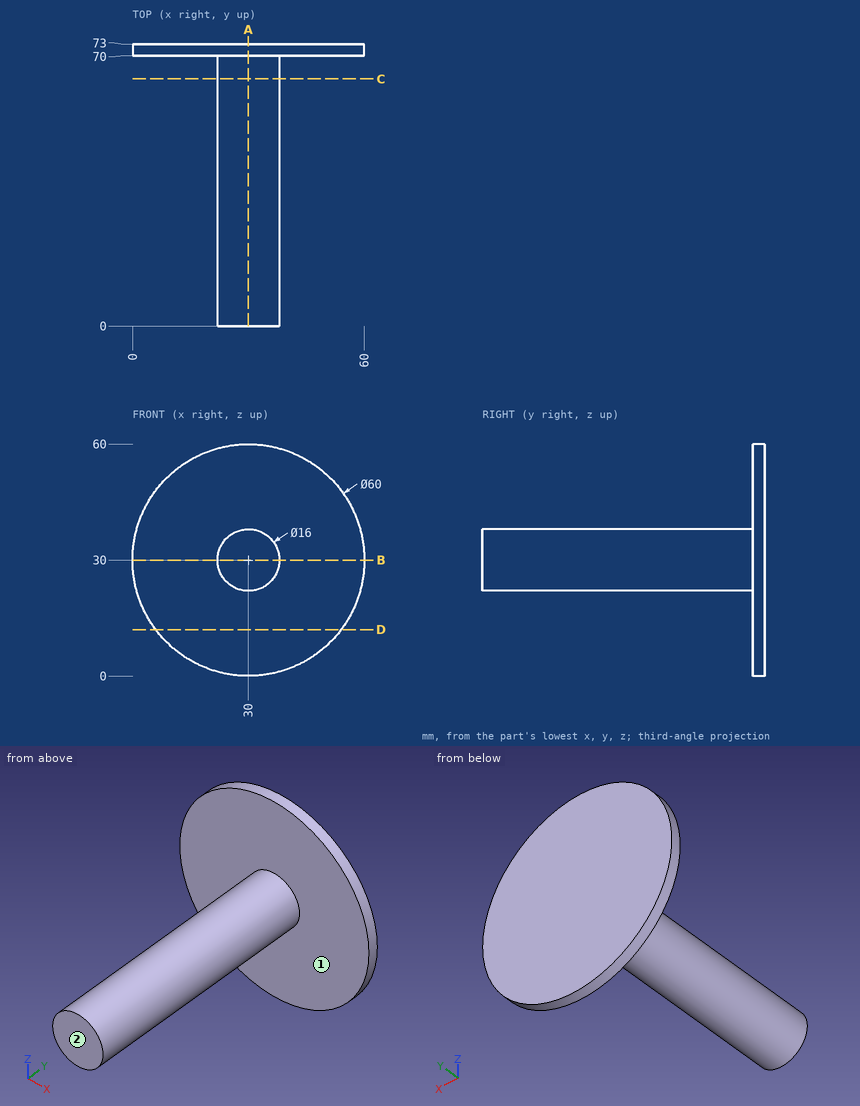
Geometry: see drawing. Coordinates: mm, zero at the bounding-box minimum. A direction names the side the tool comes from. Give positions to 0.01 mm unless a question says otherwise; leave off trailing zeros. Order: outer loops, then holes, each group sorted by start corner. A loop starts at its lowest first (then second) coordinate and runs counter-clockwise, first axis right, second up. Notation, with made-up numbers: (-29.5, 79.5) - (-15.5, 79.5) arc R9 ccw to (-15.5, 94.5) - close; hole circle Ø4 at (-35.75, 70.25). An arc over 180 degrees is marked (long way). Use a Markdown table: item, result.
(1) Section query B-B (z = 30). Output: boundary loops of the cut face in (x, y), then the cut area to 3 significant figures.
Computed values:
| item | result |
|---|---|
| outline | (0, 70) - (22, 70) - (22, 0) - (38, 0) - (38, 70) - (60, 70) - (60, 73) - (0, 73) - close |
| area | 1,300 mm2 |
(2) Pin query (flat end, axial travel): pin 1 (6 mm diameter, centred on x = 37.5, y = 50.5, fed in from +Z); pin 2 (3 mm diameter, centred on y = 38.5, z = 26.5, fed in from +X); pin 3 (10 mm diameter, centred on x = 39.5, y = 27.5, fed in from -Z). Return the tip coordinate at first contact, or that it passes through.
Computed values:
| item | result |
|---|---|
| pin 1 | stops at z = 36.61 |
| pin 2 | stops at x = 37.75 |
| pin 3 | stops at z = 23.39 |
(3) Section query A-A (x = 30). Output: boundary loops of the cut face in (y, z).
Computed values:
| item | result |
|---|---|
| outline | (0, 22) - (70, 22) - (70, 0) - (73, 0) - (73, 60) - (70, 60) - (70, 38) - (0, 38) - close |
(4) Access query for the marked faces 1 and 2. Directions: +Z, -Z, +X, -X, +Y, -Y. A direction counts if a zero-diameter tool reaches every point of the face in a straight line with its end or side. Return the directions, or none.
Computed values:
| item | result |
|---|---|
| face 1 | -Y |
| face 2 | +Z, -Z, +X, -X, -Y |
(5) Section query C-C (y = 64). Output: boundary loops of the cut face in (x, z), then the cut area to 3 significant figures.
Computed values:
| item | result |
|---|---|
| outline | circle Ø16 at (30, 30) |
| area | 201 mm2 |
(6) Section query D-D (z = 12). Output: boundary loops of the cut face in (x, y).
Computed values:
| item | result |
|---|---|
| outline | (6, 70) - (54, 70) - (54, 73) - (6, 73) - close |
(7) Line query: line 1 (Y direction, x = 28, z = 22); line 2 (X direction, y = 8, z = 26); line 3 (Z direction, x = 35, y = 62.5) (3 decimals). Output: solid intervals per line, ascending. Write a range as from..to.
Computed values:
| item | result |
|---|---|
| line 1 | y = 70..73 |
| line 2 | x = 23.07..36.93 |
| line 3 | z = 23.755..36.245 |
